Work out the finished part from the listing and answer in its coordinate system (mm). A direction names the side the tool comes from. Round coordinates to 2 decimals unless told otherwise and drop trailing zeros. Write each loop counter-clockwise with the first axis right and the second up, starting at its lowest first coordinate (ties: lowest second). Pieces come first, ordered by that corner, then holes. Notation, with made-up numbers: M 6,40.25 L 45,40.25 A10 cw 45,53.25 Z; hole C 36,30.25 d3. An arc over 180 degrees is marked long. Answer in a Markdown table with one row per item.
Autodesk Inventor part; units mm, degrees
ref_plane "YZ Plane" through (0, 0, 0) normal (1, 0, 0) x (0, 1, 0)
ref_plane "XZ Plane" through (0, 0, 0) normal (0, 1, 0) x (-1, 0, 0)
ref_plane "XY Plane" through (0, 0, 0) normal (0, 0, 1) x (1, 0, 0)
sketch "Sketch1" plane through (0, 0, 0) normal (0, 0, 1) x (1, 0, 0)
  line L0 (0, -24.5) -> (-18, -24.5)
  line L1 (-20, -22.5) -> (-20, 0)
  line L2 (-18, 2) -> (0, 2)
  line L3 (2, 0) -> (2, -22.5)
  arc A0 (-18, 2) -> (-20, 0) centre (-18, 0) ccw
  arc A1 (2, 0) -> (0, 2) centre (0, 0) ccw
  arc A2 (0, -24.5) -> (2, -22.5) centre (0, -22.5) ccw
  arc A3 (-20, -22.5) -> (-18, -24.5) centre (-18, -22.5) ccw
  dimension "d0" = 2
  dimension "d1" = 22
  dimension "d2" = 26.5
extrude "Extrusion1" add sketch "Sketch1" along normal blind 1
sketch "Sketch2" plane through (0, 0, 1) normal (0, 0, 1) x (1, 0, 0)
  line L0 (-20, 0) -> (-20, -22.5)
  line L1 (-18, -24.5) -> (0, -24.5)
  line L2 (2, -22.5) -> (2, 0)
  line L3 (0, 2) -> (-18, 2)
  line L4 (-18, 6) -> (0, 6)
  line L5 (2, 4) -> (2, -26.5)
  line L6 (0, -28.5) -> (-18, -28.5)
  line L7 (-20, -26.5) -> (-20, 4)
  arc A0 (0, -28.5) -> (2, -26.5) centre (0, -26.5) ccw
  arc A1 (-20, -26.5) -> (-18, -28.5) centre (-18, -26.5) ccw
  arc A2 (-18, 6) -> (-20, 4) centre (-18, 4) ccw
  arc A3 (2, 4) -> (0, 6) centre (0, 4) ccw
  circle A4 centre (-18, -26.5) radius 1.25
  circle A5 centre (0, 4) radius 1.25
  point P0 (0, 0)
  dimension "d5" = 2
  dimension "d6" = 4
  dimension "d7" = 4
  dimension "d8" = 2.5
  dimension "d9" = 2.5
  dimension "d18" = 34.5
  dimension "d19" = 26.5
  dimension "d20" = 22
extrude "Extrusion2" add sketch "Sketch2" along normal blind 1
chamfer "Chamfer1" distance 0.5 angle 45 8 edges at (-19.4142, 1.4142, 0) (-20, -11.25, 0) (-19.4142, -23.9142, 0) (-9, -24.5, 0) (1.4142, -23.9142, 0) (2, -11.25, 0) (1.4142, 1.4142, 0) (-9, 2, 0)
chamfer "Chamfer2" distance 0.5 angle 45 10 edges at (-20, -24.5, 1) (-19.4142, -27.9142, 1) (-9, -28.5, 1) (1.4142, -27.9142, 1) (2, -24.5, 1) (-20, 2, 1) (-19.4142, 5.4142, 1) (-9, 6, 1) (1.4142, 5.4142, 1) (2, 2, 1)
properties part number "IO-Shield-Sideplate01"
1. The part is cut by section A-A (x = -12.5). Determine the outline of the cut face in (y, z), plus the area to 3 significant figures.
Calculated:
| item | result |
|---|---|
| outline | M -28.5,1.5 L -28,1 L -24.5,1 L -24.5,0.5 L -24,0 L 1.5,0 L 2,0.5 L 2,1 L 5.5,1 L 6,1.5 L 6,2 L -28.5,2 Z |
| area | 60.5 mm² |
2. Determine the mould class of faces 4 (the flat face through (-9, -11, 2)), 5 (the cylindrical face through (-16.845, -26.021, 1.493)), 6 (the conical face through (-19.17, -27.65, 1.14)), 7 (the cylindrical face through (1.6, 1.2, 0.9)) for opening direction Y: released by +Y, released by -Y, zero draft, split by the parting line, or undercut.
Calculated:
| item | result |
|---|---|
| face 4 | zero draft |
| face 5 | undercut |
| face 6 | released by -Y |
| face 7 | released by +Y |
3. Given pin 1 (3 mm diameter, centred on x = 0, y = 4, fed in from -Z), flat-ended and moving along its own axis, determine where the tip first touches the part or whether it passes through.
Calculated:
| item | result |
|---|---|
| pin 1 | stops at z = 1 |
4. Consider line 1 along Y through (x, z) = (0, 1.4); line 2 along Y through (x, z) = (-19, 1.7); line 3 along Z through (x, y) = (-7, 4). Determine where each line is inside the solid, lowest interval first. Write a range as from..to.
Calculated:
| item | result |
|---|---|
| line 1 | y = -28.4..2.75, 5.25..5.9 |
| line 2 | y = -28.23..-27.25, -25.75..5.73 |
| line 3 | z = 1..2 |
5. A tool of negligible diameter and unlimited length cuts with its end or side. For faces 1 (the cylindrical face through (-19.6, -23.7, 0.9)), 2 (the cylindrical face through (-19.65, 1.13, 0.88)), 3 (the cylindrical face through (-0.27, 5.22, 1.49)), from which of +Z, -Z, +X, -X, +Y, -Y can it reach the whole face along a straight path? Write none if from no direction.
Calculated:
| item | result |
|---|---|
| face 1 | -Z, -X, -Y |
| face 2 | -Z, -X, +Y |
| face 3 | +Z, -Z |
